Check sheet for the drawn part. Datum: minimum x, y, z corner. Units: mm. A direction names the side the tool comes from. Give positions to 0.01 mm unless a question says otherwise; leave off trailing zeros. Loops run counter-clockwise (first coordinate to the right, second up) from the corner with the lowest first, then second, coordinate; pieces in that order, holes last. Notation, with made-up numbers: (-25, 17) - (6, 17) arc R5 ccw to (6, 26) - close; hole circle Ø9 at (28.5, 80). An arc over 180 degrees is marked (long way). Use one line per item in the form item = value.
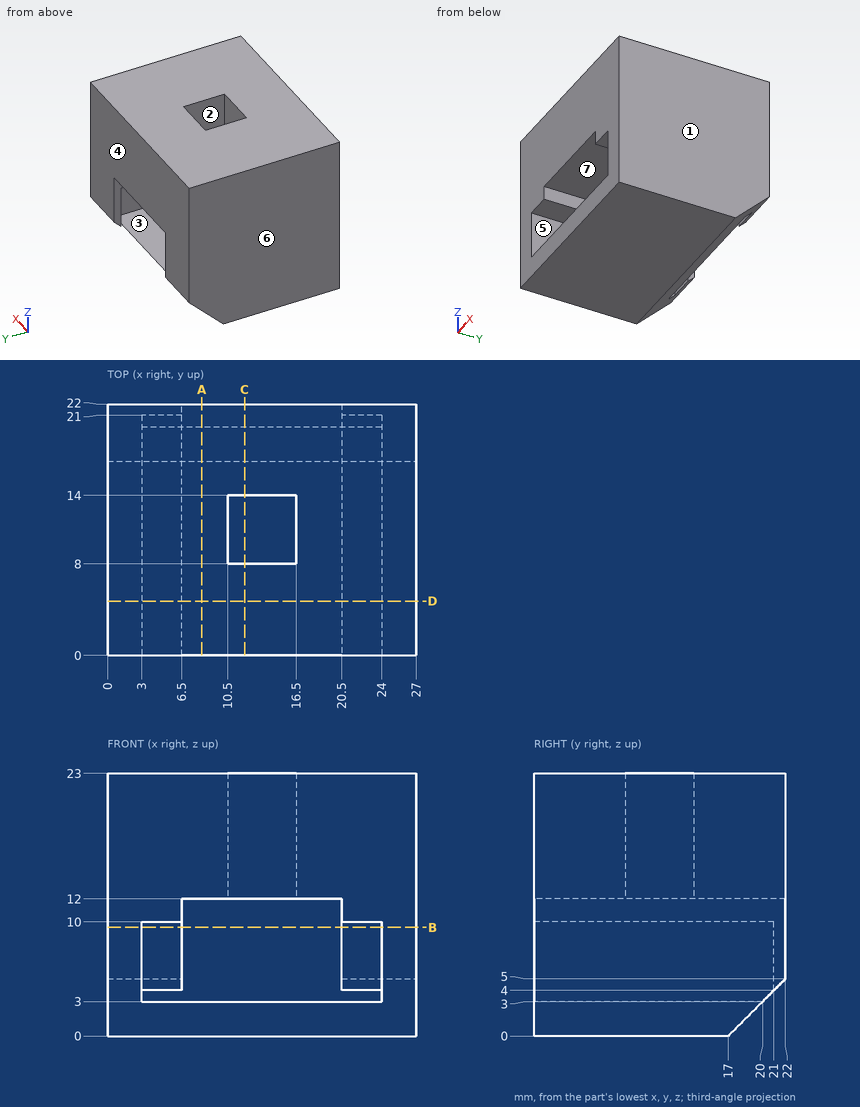
1. Section check A-A, the plane x = 8.25. Record the cut outline in (y, z).
Result set:
outline = (0, 0) - (17, 0) - (20, 3) - (0, 3) - close; (0, 12) - (22, 12) - (22, 23) - (0, 23) - close
2. Section check B-B, the plane z = 9.5. Record the cut outline in (x, y), then the cut area to 3 significant figures.
Result set:
outline = (0, 0) - (3, 0) - (3, 21) - (6.5, 21) - (6.5, 22) - (0, 22) - close; (20.5, 21) - (24, 21) - (24, 0) - (27, 0) - (27, 22) - (20.5, 22) - close
area = 139 mm²
3. Section check D-D, the plane y = 4.75. Record the cut outline in (x, z), then the cut area to 3 significant figures.
Result set:
outline = (0, 0) - (27, 0) - (27, 23) - (0, 23) - close; hole (3, 3) - (24, 3) - (24, 10) - (20.5, 10) - (20.5, 12) - (6.5, 12) - (6.5, 10) - (3, 10) - close
area = 446 mm²
4. Depth check by flat-ended pin: pin 1 Ø1 at (x, z) = (5, 7) entering from -Y. Enter the tip coordinate at first touch or a pass-through.
Result set:
pin_1 = 21
5. Section check C-C, the plane x = 12. Record the cut outline in (y, z), then the cut area to 4 significant figures.
Result set:
outline = (0, 0) - (17, 0) - (20, 3) - (0, 3) - close; (0, 12) - (8, 12) - (8, 23) - (0, 23) - close; (14, 12) - (22, 12) - (22, 23) - (14, 23) - close
area = 231.5 mm²
6. Scan lines: probe 1 along X at (y, z) = (12, 18.75); probe 2 along X at (y, z) = (13.75, 4.5); probe 3 along Z at (x, y) = (7.25, 9.75). Record each from-to range of solid material in increasing order.
Result set:
probe_1 = 0 to 10.5, 16.5 to 27
probe_2 = 0 to 3, 24 to 27
probe_3 = 0 to 3, 12 to 23
7. Draft check along X on the marked faces 1, 2, 3 and 4. Enter one of: released by +X, released by -X, zero draft, split by the parting line, or undercut.
Result set:
face_1 = released by +X
face_2 = undercut
face_3 = undercut
face_4 = zero draft
8. Tool access check on the marked faces 5, 6 and 7. Record the directions out of +Z, -Z, +X, -X, +Y, -Y that give a thin tool (end or side, any length) a straight path to the whole face; none if there is none.
Result set:
face_5 = -Y
face_6 = +Z, -Z, -X, +Y, -Y
face_7 = +Y, -Y
